For this review, take the finished solid that the model builds, in its own axes (mm). Face numbers are marked on the shaded views. A direction names the side the tool comes from. Give positions to 0.01 mm unless a question says otherwise; leave off trailing zeros. Loops run counter-clockwise (first coordinate to the right, second up) from the corner with the lowest first, then second, coordinate; pieces in that order, holes last. Notation, with made-up numbers: M 16,-32 L 30,-32 A13 cw 30,-20 Z; hole C 62.25,-32.5 d9. An arc over 180 degrees is marked long. Use CSV: the item, a comma, the result in double quotes. Start each with the question number.
1. Insertion check: P1, Ø6, axis at x = -15, z = 534, coming from the +Y side; P2, Ø2.5, axis at x = 15, z = 534, coming from the +Y side; P3, Ø4.5, axis at x = 20.5, y = 0, coming from the +Z side. Each pin has a flat end and moves straight along its axis. Give the tip position at first contact, or say it passes through.
2. The part is to be moulded in two halves that separate along X. For the marked faces 3, 4 and 5, say which applies: pulls with the +X half, pulls with the -X half, needs draft (parallel to the pull), parting line crosses it, or undercut.
3. Tool access review of the marked faces 1 and 2: name each direction out of +Z, -Z, +X, -X, +Y, -Y from which nothing blocks a thin tool from reaching the whole face with its end or side.
4. Take a section at C-C, the plane z = 539. Write out the cut boundary in (x, y), and give its area (3 significant figures).
5. To check wall thickness, follow line 1 (Y direction, x = -10.25, z = 523.7); line 2 (X direction, y = -31, z = 534); line 3 (Y direction, x = -5, z = 539). State the ranges of each line that lie inside material, in increasing order. Write a range as [from, to].
6. Take a section at B-B, the plane y = 0. Write out the cut boundary in (x, z), and give its area (3 significant figures).
7. Take a section at A-A, the plane x = 0. Write out the cut boundary in (y, z).
8. Take a section at D-D, the plane x = 10.25. Write out the cut boundary in (y, z), and give its area (3 significant figures).
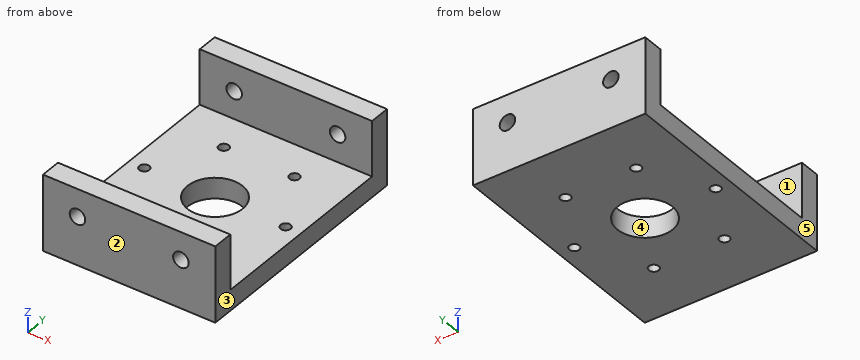
from build123d import *

# Parameters (mm, degrees)
REPISA_START                   = 520
SK_REPISA_W                    = 50
SK_REPISA_H                    = 69
REPISA_DEPTH                   = 6
CENTRO_MOTOR_START             = 520
SK_CENTRO_MOTOR_R              = 8
CENTRO_MOTOR_DEPTH             = 6
PASANTES_M2_5_ESTATOR_J6_START = 520
SK_PASANTES_M2_5_ESTATOR_J6_R  = 1.45
PASANTES_M2_5_ESTATOR_J6_DEPTH = 6
PESTANAS_START                 = 526
SK_PESTANAS_W                  = 50
SK_PESTANAS_H                  = 6
PESTANAS_DEPTH                 = 16
PASANTES_M4_PESTANAS_START     = -34.5
SK_PASANTES_M4_PESTANAS_R      = 2.25
PASANTES_M4_PESTANAS_DEPTH     = 69


with BuildPart() as part:
    # Sk_Repisa → Repisa (new body)
    with BuildSketch(Plane.XY.offset(REPISA_START)):
        Rectangle(SK_REPISA_W, SK_REPISA_H)
    extrude(amount=REPISA_DEPTH)

    # Sk_Centro_motor → Centro_motor (cut)
    with BuildSketch(Plane.XY.offset(CENTRO_MOTOR_START)):
        Circle(SK_CENTRO_MOTOR_R)
    extrude(amount=CENTRO_MOTOR_DEPTH, mode=Mode.SUBTRACT)

    # Sk_Pasantes_M2-5_estator_J6 → Pasantes_M2-5_estator_J6 (cut)
    with BuildSketch(Plane.XY.offset(PASANTES_M2_5_ESTATOR_J6_START)):
        with Locations((20.5, 0)):
            Circle(SK_PASANTES_M2_5_ESTATOR_J6_R)
        with Locations((10.25, 17.753520778)):
            Circle(SK_PASANTES_M2_5_ESTATOR_J6_R)
        with Locations((-10.25, 17.753520778)):
            Circle(SK_PASANTES_M2_5_ESTATOR_J6_R)
        with Locations((-20.5, 0)):
            Circle(SK_PASANTES_M2_5_ESTATOR_J6_R)
        with Locations((-10.25, -17.753520778)):
            Circle(SK_PASANTES_M2_5_ESTATOR_J6_R)
        with Locations((10.25, -17.753520778)):
            Circle(SK_PASANTES_M2_5_ESTATOR_J6_R)
    extrude(amount=PASANTES_M2_5_ESTATOR_J6_DEPTH, mode=Mode.SUBTRACT)

    # Sk_Pestanas → Pestanas (add)
    with BuildSketch(Plane.XY.offset(PESTANAS_START)):
        with Locations((0, 31.5)):
            Rectangle(SK_PESTANAS_W, SK_PESTANAS_H)
        with Locations((0, -31.5)):
            Rectangle(SK_PESTANAS_W, SK_PESTANAS_H)
    extrude(amount=PESTANAS_DEPTH)

    # Sk_Pasantes_M4_pestanas → Pasantes_M4_pestanas (cut)
    with BuildSketch(Plane(origin=(0, 0, 0), x_dir=(1, 0, 0), z_dir=(0, 1, 0)).offset(PASANTES_M4_PESTANAS_START)):
        with Locations(Location((-15, -534, 0), (0, 0, 270))):
            Circle(SK_PASANTES_M4_PESTANAS_R)
        with Locations(Location((15, -534, 0), (0, 0, 270))):
            Circle(SK_PASANTES_M4_PESTANAS_R)
    extrude(amount=PASANTES_M4_PESTANAS_DEPTH, mode=Mode.SUBTRACT)


solid = part.part
Result set:
1,P1,"y = 34.5"
1,P2,"through"
1,P3,"z = 526"
2,face 3,"pulls with the +X half"
2,face 4,"undercut"
2,face 5,"pulls with the -X half"
3,face 1,"+Z, +X, -X"
3,face 2,"+Z, -Z, +X, -X, -Y"
4,outline,"M -25,-34.5 L 25,-34.5 L 25,-28.5 L -25,-28.5 Z; M -25,28.5 L 25,28.5 L 25,34.5 L -25,34.5 Z"
4,area,"600 mm2"
5,line 1,"[-34.5, -19.2], [-16.3, 16.3], [19.2, 34.5]"
5,line 2,"[-25, -17.25], [-12.75, 12.75], [17.25, 25]"
5,line 3,"[-34.5, -28.5], [28.5, 34.5]"
6,outline,"M -25,520 L -21.95,520 L -21.95,526 L -25,526 Z; M -19.05,520 L -8,520 L -8,526 L -19.05,526 Z; M 8,520 L 19.05,520 L 19.05,526 L 8,526 Z; M 21.95,520 L 25,520 L 25,526 L 21.95,526 Z"
6,area,"169 mm2"
7,outline,"M -34.5,520 L -8,520 L -8,526 L -28.5,526 L -28.5,542 L -34.5,542 Z; M 8,520 L 34.5,520 L 34.5,542 L 28.5,542 L 28.5,526 L 8,526 Z"
8,outline,"M -34.5,520 L -19.2,520 L -19.2,526 L -28.5,526 L -28.5,542 L -34.5,542 Z; M -16.3,520 L 16.3,520 L 16.3,526 L -16.3,526 Z; M 19.2,520 L 34.5,520 L 34.5,542 L 28.5,542 L 28.5,526 L 19.2,526 Z"
8,area,"571 mm2"
